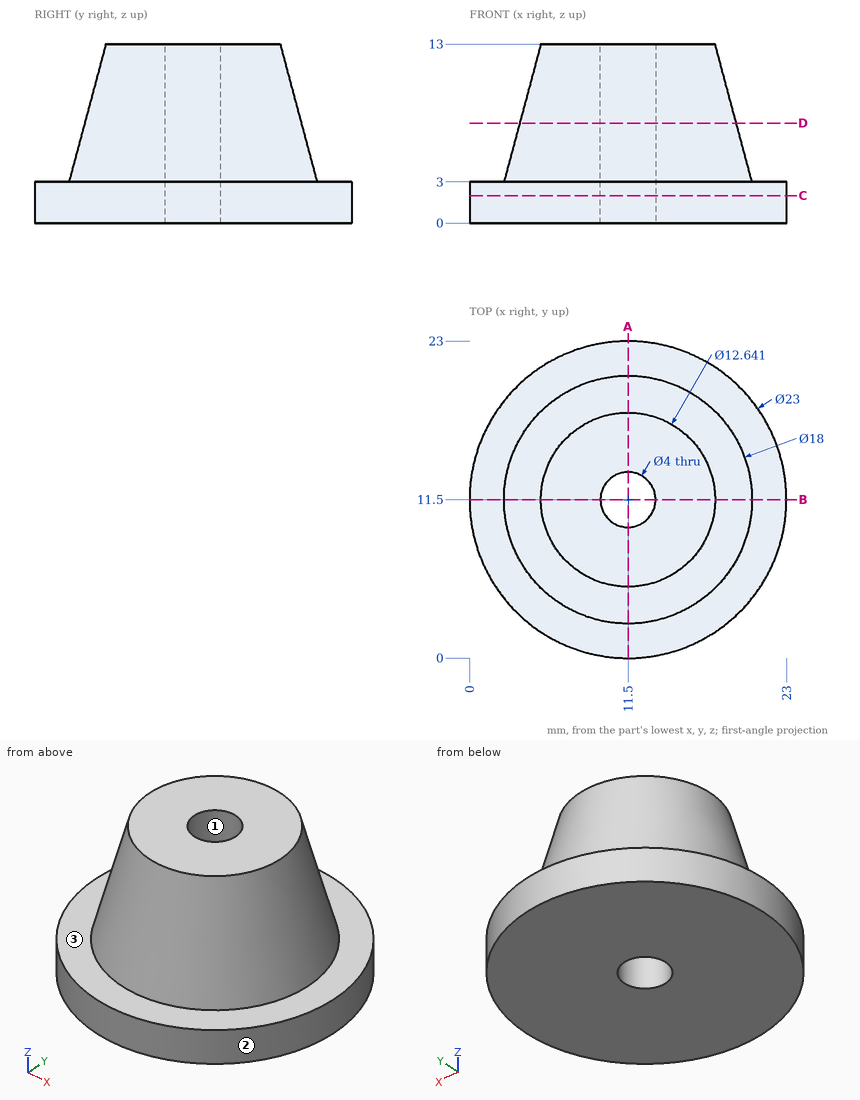
Print and shaded views of the part. All mm, measured from the part's lowest x, y and z. Give positions to 0.01 mm unless a question says otherwise; leave off trailing zeros. Loops run counter-clockwise (first coordinate to the right, second up) from the corner with the lowest first, then second, coordinate; pieces in that order, holes last.
1) Saw through at D-D (z = 7.25). Write the cut outline in (x, y), plus the area to 3 significant figures.
2) Wall check: line 1 (Y direction, x = 11.5, z = 10.75); line 2 (Z direction, x = 13, y = 21.75); line 3 (X direction, y = 11, z = 0.5). Give the ranges that are in metal, low to high.
3) Saw through at C-C (z = 2). Write the cut outline in (x, y), plus the area to 3 significant figures.
4) Pull direction X, two halves, no side cores. Call the marked faces 1, 2 and 3: +X half, -X half, draft (parallel to the pull), parting line (faces both ways), or undercut.
5) Saw through at A-A (x = 11.5). Write the cut outline in (y, z), plus the area to 3 significant figures.
6) Flat gauge pins, fed straight in: pin 1 Ø4 at (y, z) = (12.5, 1.5) entering from -X; pin 2 Ø4 at (y, z) = (2.5, 2) entering from -X; pin 3 Ø4 at (y, z) = (3, 1.5) entering from +X; pin 4 Ø3 at (y, z) = (15, 5.5) entering from -X. Where does each tip first touch, or does it go through?
Answer block:
1. outline: circle Ø15.72 at (11.5, 11.5); hole circle Ø4 at (11.5, 11.5)
1. area: 182 mm2
2. line 1: y = 4.58 to 9.5, 13.5 to 18.42
2. line 2: z = 0 to 3
2. line 3: x = 0.01 to 9.56, 13.44 to 22.99
3. outline: circle Ø23 at (11.5, 11.5); hole circle Ø4 at (11.5, 11.5)
3. area: 403 mm2
4. face 1: undercut
4. face 2: parting line
4. face 3: draft
5. outline: (0, 0) - (9.5, 0) - (9.5, 13) - (5.18, 13) - (2.5, 3) - (0, 3) - close; (13.5, 0) - (23, 0) - (23, 3) - (20.5, 3) - (17.82, 13) - (13.5, 13) - close
5. area: 170 mm2
6. pin 1: stops at x = 0
6. pin 2: stops at x = 2.38
6. pin 3: stops at x = 20.99
6. pin 4: stops at x = 3.24
